```python
from build123d import *

# Parameters (mm, degrees)
SKETCH2_ONE_SIDE_W  = 4
SKETCH2_ONE_SIDE_H  = 12.25
BOSS_EXTRUDE1_DEPTH = 4
SKETCH4_R           = 0.6
CUT_EXTRUDE1_DEPTH  = 0.2
SKETCH5_R           = 11
CUT_EXTRUDE2_DEPTH  = 4
SKETCH6_R           = 3
CUT_EXTRUDE3_DEPTH  = 11


with BuildPart() as part:
    # Sketch2 one side → Revolve3 (revolve)
    with BuildSketch(Plane(origin=(0, 0, 0), x_dir=(0, 0, -1), z_dir=(1, 0, 0))):
        Polygon((12.3, 0), (12.3, 8.15), (0, 7.65), (0, 0), align=None)
        Polygon((15.3, 0), (15.3, 12.25), (12.3, 8.15), (12.3, 0), align=None)
        with Locations((17.3, 6.125)):
            Rectangle(SKETCH2_ONE_SIDE_W, SKETCH2_ONE_SIDE_H)
    revolve(axis=Axis((0, 0, 0), (0, 0, -1)))

    # Sketch3 → Boss-Extrude1 (add)
    with BuildSketch(Plane(origin=(0, 0, -19.3), x_dir=(-1, 0, 0), z_dir=(0, 0, -1))):
        Polygon((0, 13.98), (1.154700538, 11.98), (-1.154700538, 11.98), align=None)
    extrude(amount=-BOSS_EXTRUDE1_DEPTH)

    # Sketch4 → Cut-Extrude1 (cut)
    with BuildSketch(Plane.XY):
        with Locations((0, 5.15)):
            Circle(SKETCH4_R)
    extrude(amount=-CUT_EXTRUDE1_DEPTH, mode=Mode.SUBTRACT)

    # Sketch5 → Cut-Extrude2 (cut)
    with BuildSketch(Plane(origin=(0, 0, -19.3), x_dir=(-1, 0, 0), z_dir=(0, 0, -1))):
        Circle(SKETCH5_R)
    extrude(amount=-CUT_EXTRUDE2_DEPTH, mode=Mode.SUBTRACT)

    # Sketch6 → Cut-Extrude3 (cut)
    with BuildSketch(Plane(origin=(0, 0, -15.3), x_dir=(-1, 0, 0), z_dir=(0, 0, -1))):
        Circle(SKETCH6_R)
    extrude(amount=-CUT_EXTRUDE3_DEPTH, mode=Mode.SUBTRACT)


solid = part.part
```
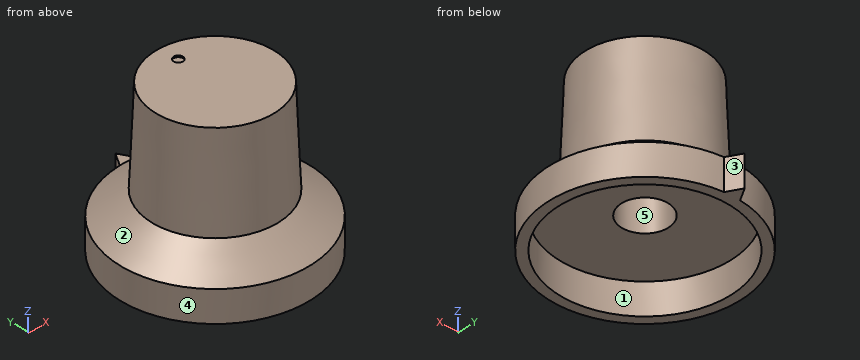
Model file for the job. Use its own axes, mm. Face numbers are marked on the shaded views. A direction names the side the tool comes from. Coordinates: 2 decimals unless noted, no trailing zeros. Loops run counter-clockwise (first coordinate to the right, second up) from the corner with the lowest first, then second, coordinate; pieces in that order, holes last. Notation, with made-up numbers: (25.25, 7.5) - (30.25, 7.5) arc R22 ccw to (30.25, 25.5) - close; hole circle Ø9 at (49, 31). An arc over 180 degrees is marked (long way). Write item = value, one per line. Start each with the question number.
Item 1: Saw through at B-B, the plane z = -5.5. List the corners of the cut face in (x, y), then the cut area to 3 significant figures.
Item 2: Drop flat-ended pins along their axis: pin 1 Ø2 at (x, z) = (-2, -9) entering from +Y; pin 2 Ø1.5 at (x, y) = (5.5, -6) entering from -Z; pin 3 Ø1.8 at (x, y) = (-1.5, 1) entering from -Z. Give the stop position or say it passes through.
Item 3: Saw through at A-A, the plane y = 0. List the corners of the cut face in (x, z), then the cut area to 3 significant figures.
Item 4: 3-axis set-ups, long thin cutter, end or side, ignore diameter. For the marked faces 1 and 2: which of +Z, -Z, +X, -X, +Y, -Y reach the whole face in a straight line?
Item 5: Saw through at C-C, the plane z = -2.5. List the corners of the cut face in (x, y).
Item 6: Wall check: probe 1 along Y at (x, z) = (0, -0.05); probe 2 along Z at (x, y) = (-2, -7); probe 3 along Y at (x, z) = (0.75, -16). Give the ranges that are in metal, low to high. Write a range as [from, to].
Item 7: Pull direction Y, two halves, no side cores. Call the marked faces 3, 4 and 5: +Y half, -Y half, draft (parallel to the pull), parting line (faces both ways), or undercut.
Answers:
q1.outline = circle Ø15.75 at (0, 0); hole circle Ø6 at (0, 0)
q1.area = 166 mm2
q2.pin_1 = 7.96
q2.pin_2 = -15.3
q2.pin_3 = -4.3
q3.outline = (-12.25, -19.3) - (-11, -19.3) - (-11, -15.3) - (-3, -15.3) - (-3, -4.3) - (3, -4.3) - (3, -15.3) - (11, -15.3) - (11, -19.3) - (12.25, -19.3) - (12.25, -15.3) - (8.15, -12.3) - (7.65, 0) - (-7.65, 0) - (-8.15, -12.3) - (-12.25, -15.3) - close
q3.area = 200 mm2
q4.face_1 = -Z
q4.face_2 = +Z
q5.outline = circle Ø15.5 at (0, 0)
q6.probe_1 = [-7.65, 4.55], [5.75, 7.65]
q6.probe_2 = [-15.3, 0]
q6.probe_3 = [-12.23, -10.97], [10.97, 12.68]
q7.face_3 = +Y half
q7.face_4 = parting line
q7.face_5 = undercut
